Source: CAD feature listing. Evaluate the final solid. Frame: model axes, mm. A direction names the side the tool comes from. Coordinates: 2 decimals unless noted, no trailing zeros. Order: outer loops, then holes, each group sorted by start corner. A loop starts at its lowest first (then second) coordinate and runs counter-clockwise, first axis right, second up.
```python
from build123d import *

# Parameters (mm, degrees)
SKETCH1_R           = 1.6
BOSS_EXTRUDE1_DEPTH = 5
SKETCH2_W           = 6
SKETCH2_H           = 50
BOSS_EXTRUDE2_DEPTH = 32
SKETCH3_R           = 2.7
CUT_EXTRUDE1_DEPTH  = 7
SKETCH4_R           = 8
CUT_EXTRUDE2_DEPTH  = 3
CUT_EXTRUDE3_DEPTH  = 68.692277038


with BuildPart() as part:
    # Sketch1 → Boss-Extrude1 (new body)
    with BuildSketch(Plane.XY):
        with BuildLine():
            Line((-11, -9.487882213), (11, -9.487882213))
            ThreePointArc((11, -9.487882213), (14.535533906, -10.952348307), (16, -14.487882213))
            Line((16, -14.487882213), (16, -36.487882213))
            ThreePointArc((16, -36.487882213), (14.535533906, -40.023416119), (11, -41.487882213))
            Line((11, -41.487882213), (-11, -41.487882213))
            ThreePointArc((-11, -41.487882213), (-14.535533906, -40.023416119), (-16, -36.487882213))
            Line((-16, -36.487882213), (-16, -14.487882213))
            ThreePointArc((-16, -14.487882213), (-14.535533906, -10.952348307), (-11, -9.487882213))
        make_face()
        with Locations((11.66726189, -13.820620324)):
            Circle(SKETCH1_R, mode=Mode.SUBTRACT)
        with Locations((11.66726189, -37.155144103)):
            Circle(SKETCH1_R, mode=Mode.SUBTRACT)
        with Locations((-11.66726189, -37.155144103)):
            Circle(SKETCH1_R, mode=Mode.SUBTRACT)
        with Locations((-11.66726189, -13.820620324)):
            Circle(SKETCH1_R, mode=Mode.SUBTRACT)
    extrude(amount=-BOSS_EXTRUDE1_DEPTH)

    # Sketch2 → Boss-Extrude2 (add)
    with BuildSketch(Plane(origin=(0, -9.487882213, 0), x_dir=(1, 0, 0), z_dir=(0, 1, 0))):
        with Locations((0, 25)):
            Rectangle(SKETCH2_W, SKETCH2_H)
    extrude(amount=-BOSS_EXTRUDE2_DEPTH)

    # Sketch3 → Cut-Extrude1 (cut)
    with BuildSketch(Plane.ZY.offset(3)):
        with Locations((-34, -25.487882213)):
            Circle(SKETCH3_R)
    extrude(amount=-CUT_EXTRUDE1_DEPTH, mode=Mode.SUBTRACT)

    # Sketch4 → Cut-Extrude2 (cut)
    with BuildSketch(Plane.XY):
        with Locations((0, -25.487882213)):
            Circle(SKETCH4_R)
    extrude(amount=-CUT_EXTRUDE2_DEPTH, mode=Mode.SUBTRACT)

    # Sketch7 → Cut-Extrude3 (cut, through all)
    with BuildSketch(Plane.ZY.offset(3)):
        with BuildLine():
            Line((-34, -9.487882213), (-52.373766184, -9.487882213))
            Line((-52.373766184, -9.487882213), (-52.373766184, -41.487882213))
            Line((-52.373766184, -41.487882213), (-34, -41.487882213))
            ThreePointArc((-34, -41.487882213), (-50, -25.487882213), (-34, -9.487882213))
        make_face()
    extrude(amount=-CUT_EXTRUDE3_DEPTH, mode=Mode.SUBTRACT)


solid = part.part
```
Q1. Section query C-C on x = -5. Output: boundary loops of the cut face in (y, z).
Solutions:
outline: (-41.49, -5) - (-9.49, -5) - (-9.49, 0) - (-19.24, 0) - (-19.24, -3) - (-31.73, -3) - (-31.73, 0) - (-41.49, 0) - close
Q2. Section query B-B on y = -11.5. Output: boundary loops of the cut face in (x, z), plus the area to 3 significant figures.
Solutions:
outline: (-15.01, -5) - (-3, -5) - (-3, -41.77) - (3, -41.77) - (3, -5) - (15.01, -5) - (15.01, 0) - (-15.01, 0) - close
area: 371 mm2
Q3. Section query A-A on x = 0. Output: boundary loops of the cut face in (y, z).
Solutions:
outline: (-41.49, -34) arc R16 ccw to (-9.49, -34) - (-9.49, 0) - (-17.49, 0) - (-17.49, -3) - (-33.49, -3) - (-33.49, 0) - (-41.49, 0) - close; hole circle Ø5.4 at (-25.49, -34)
Q4. Section query D-D on z = -14. Output: boundary loops of the cut face in (x, y).
Solutions:
outline: (-3, -41.49) - (3, -41.49) - (3, -9.49) - (-3, -9.49) - close
Q5. Material intervals for line 1 along X through (y, z) = (-14, -38); line 2 along X through (y, z) = (-38, -4.5); line 3 along Z through (x, y) = (-8, -35.5), sorted ascending.
Solutions:
line 1: x = -3 to 3
line 2: x = -15.77 to -13.03, -10.31 to 10.31, 13.03 to 15.77
line 3: z = -5 to 0
Q6. Pull-direction query (Y, two-part tool) for faces 1 (the cylindrical face through (-10.807, -35.806, -2.465)), 2 (the flat face through (0, -41.488, -13)), 3 (the cylindrical face through (14.496, -10.914, -2.465)); classes: pulls with the +Y half, pulls with the -Y half, needs draft (parallel to the pull), parting line crosses it, or undercut.
Solutions:
face 1: undercut
face 2: pulls with the -Y half
face 3: pulls with the +Y half
Q7. Set-up query: faces 4 (the flat face through (-16, -26, -2)), 5 (the cylindrical face through (-14.57, -10.99, -2.46)), 6 (the flat face through (3, -25, -27)), 7 (the flat face through (-3, -25, -27)), 8 (the flat face through (0, -25, -3)). Return all of +Z, -Z, +X, -X, +Y, -Y with unobstructed straight access to the full face (end or side cutting, diameter ignored); none if empty.
Solutions:
face 4: +Z, -Z, -X, +Y, -Y
face 5: +Z, -Z, -X, +Y
face 6: -Z, +X, +Y, -Y
face 7: -Z, -X, +Y, -Y
face 8: +Z
Q8. Pin query (flat end, axial travel): P1, Ø8, axis at y = -17.5, z = -44.5, coming from the +X side; P2, Ø8.5, axis at y = -25.49, z = -34, coming from the -X side; P3, Ø10, axis at x = -4.5, y = -32, coming from the +Z side; P4, Ø4, axis at x = 9, y = -27, coming from the -Z side. Return the tip coordinate at first contact, or that it passes through.
Solutions:
P1: stops at x = 3
P2: stops at x = -3
P3: stops at z = 0
P4: stops at z = -5
